Could you check a few things on this drawing? It's one solid part, dimensions in mm from its lowest x, y, z. A direction names the side the tool comes from. Give positions to 0.01 mm unless a question says otherwise; leave off trailing zeros. Write each loop counter-clockwise with the first axis right and the second up, starting at its lowest first coordinate (ties: lowest second). Pieces come first, ordered by that corner, then holes. Notation, with made-up numbers: (63.25, 69) -> (74.25, 69) arc R16 cw to (74.25, 89) -> close; hole circle Ø1 at (31.25, -19.75). An arc over 180 degrees is marked (long way). Answer as CSV lines item,"result". Start each with the question number.
1. If we section it at C-C on y = 1.45: Write out the boundary of the cut face in (x, z).
2. I need wall thicknesses on line 1 (Z direction, x = 8, y = 1.2); line 2 (X direction, y = 2.25, z = 4.5); line 3 (X direction, y = 0.6, z = 7.75). Which ranges of each line are inside material? Lowest first, please. Write a range as [from, to].
3. On a 3-axis mill with a long thin cutter (end or side, diameter ignored), from which of +Z, -Z, +X, -X, +Y, -Y can I reach the whole of each face in a straight line? I mean the marked faces 1 and 2. Say none if no direction works.
4. If we section it at D-D on z = 1.25: Write out the boundary of the cut face in (x, y).
5. If we section it at A-A on z = 2.75: Write out the boundary of the cut face in (x, y).
6. If we mould it in two halves opening along Z, with no side actions, what happens to the marked faces 3, 4, 5 and 6? For each: pulls with the +Z half, pulls with the -Z half, needs draft (parallel to the pull), parting line crosses it, or undercut.
7. If we section it at B-B on x = 13.25: Write out the boundary of the cut face in (y, z), plus the area to 3 significant figures.
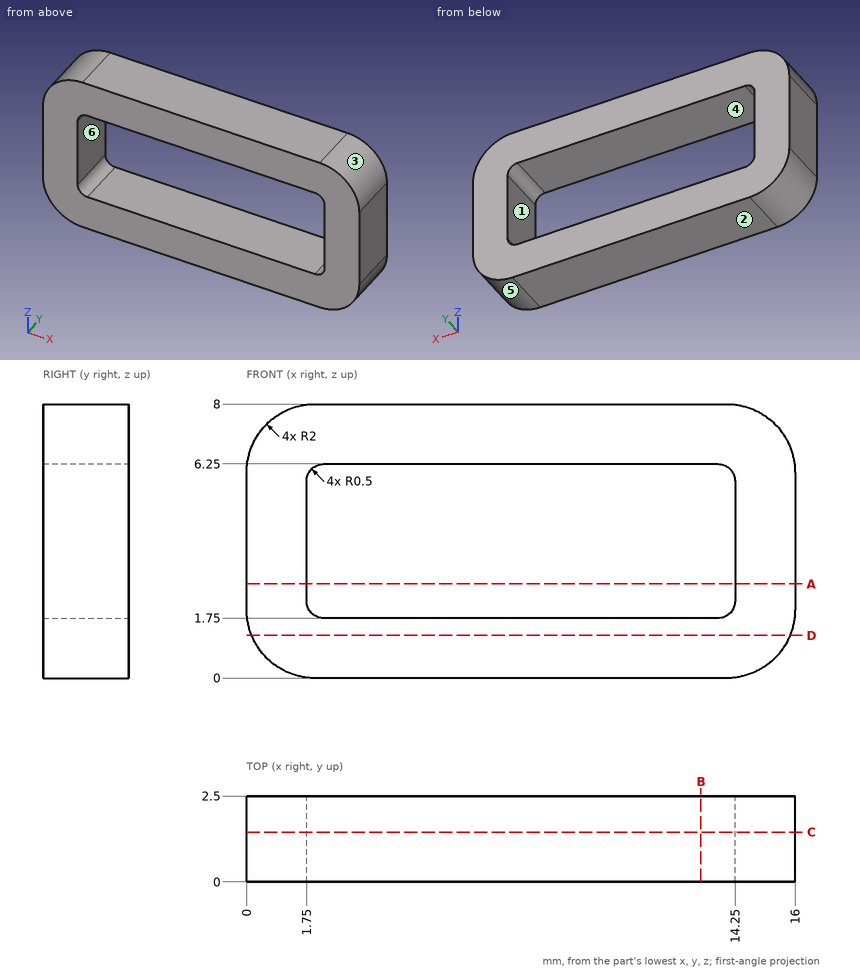
Computed values:
1,outline,"(0, 2) arc R2 ccw to (2, 0) -> (14, 0) arc R2 ccw to (16, 2) -> (16, 6) arc R2 ccw to (14, 8) -> (2, 8) arc R2 ccw to (0, 6) -> close; hole (1.75, 2.25) arc R0.5 ccw to (2.25, 1.75) -> (13.75, 1.75) arc R0.5 ccw to (14.25, 2.25) -> (14.25, 5.75) arc R0.5 ccw to (13.75, 6.25) -> (2.25, 6.25) arc R0.5 ccw to (1.75, 5.75) -> close"
2,line 1,"z = [0, 1.75], [6.25, 8]"
2,line 2,"x = [0, 1.75], [14.25, 16]"
2,line 3,"x = [1.03, 14.97]"
3,face 1,"+Y, -Y"
3,face 2,"-Z, +X, -X, +Y, -Y"
4,outline,"(0.15, 0) -> (15.85, 0) -> (15.85, 2.5) -> (0.15, 2.5) -> close"
5,outline,"(0, 0) -> (1.75, 0) -> (1.75, 2.5) -> (0, 2.5) -> close; (14.25, 0) -> (16, 0) -> (16, 2.5) -> (14.25, 2.5) -> close"
6,face 3,"pulls with the +Z half"
6,face 4,"undercut"
6,face 5,"pulls with the -Z half"
6,face 6,"undercut"
7,outline,"(0, 0) -> (2.5, 0) -> (2.5, 1.75) -> (0, 1.75) -> close; (0, 6.25) -> (2.5, 6.25) -> (2.5, 8) -> (0, 8) -> close"
7,area,"8.75 mm2"
